Part model, mm, in its own coordinate system. A direction names the side the tool comes from. Round coordinates to 2 decimals unless told otherwise and drop trailing zeros. Write each loop counter-clockwise with the first axis right and the second up, starting at its lowest first coordinate (ties: lowest second). Pieces come first, ordered by that corner, then holes. Notation, with made-up numbers: M 60.5,30.25 L 65.5,30.25 A16 cw 65.5,51.25 Z; hole C -20,49.25 d3. An arc over 180 degrees is marked long. Answer as a JSON object with one key per item and string values. Group by question number.
1. Drop flat-ended pins along their axis: pin 1 (1.5 mm diameter, centred on x = -6, y = -5.5, fed in from +Z); pin 2 (2.5 mm diameter, centred on y = 44.5, z = 10.5, fed in from -X); pin 3 (5 mm diameter, centred on x = -15, z = 10.5, fed in from +Y). Give the stop position or say it passes through.
2. Band-saw the part on B-B, the plane x = -12.25. Write the cut outline in (y, z).
3. Two-plate mould, pull along X, no slides. Class faces 1 (the face through (-17.586, 131.112, 6.409)), 2 (the face through (0.23, 132.16, 6.41)), 3 (the face through (-5.654, 115.116, 6.409)): +X half, -X half, draft (parallel to the pull), parting line (faces both ways), or undercut.
4. Drill centre lines: line 1 (X direction, y = 0.5, z = 6); line 2 (Y direction, x = -5, z = 2.75); line 3 (Y direction, x = -7.25, z = 9.5). Where is each one in solid material? Low to high. Write a range as from..to.
5. Band-saw the part on D-D, the plane y = 104.5. Write the cut outline in (x, z).
6. Band-saw the part on A-A, the plane z = 3. Write the cut outline in (x, y), plus the area to 3 significant figures.
7. Band-saw the part on C-C, the plane y = 13.5. Write the cut outline in (x, z).
8. Which spindle directions (+Z, -Z, +X, -X, +Y, -Y) get a long thin tool onto all of the face, cutting with end or side? Do faces 4 (the face through (-11.556, 158.073, 6.409)), 5 (the face through (-5.439, 87.636, 9.056)), 6 (the face through (-14.329, 36, 6)). Say none if no direction does.
from build123d import *

# Parameters (mm, degrees)
SKETCH1_R      = 2.5
EXTRUDE1_DEPTH = 13
EXTRUDE2_DEPTH = 8


with BuildPart() as part:
    # Sketch1 → Extrude1 (new body)
    with BuildSketch(Plane.XY):
        with BuildLine():
            Line((-14.328597561, 112.637649389), (-14.328597561, -42.362350611))
            ThreePointArc((-14.328597561, -42.362350611), (-5.328597561, -51.362350611), (3.671402439, -42.362350611))
            Line((3.671402439, -42.362350611), (3.671402439, 112.637649389))
            ThreePointArc((3.671402439, 112.637649389), (3.534672216, 114.200482988), (3.128636026, 115.715830679))
            Line((3.128636026, 115.715830679), (-2.753580135, 149.07553625))
            ThreePointArc((-2.753580135, 149.07553625), (-11.753580135, 158.07553625), (-20.753580135, 149.07553625))
            Line((-20.753580135, 149.07553625), (-14.328597561, 112.637649389))
        make_face()
        with Locations((-5.328597561, 112.637649389)):
            Circle(SKETCH1_R, mode=Mode.SUBTRACT)
        with Locations((-5.328597561, -42.362350611)):
            Circle(SKETCH1_R, mode=Mode.SUBTRACT)
        with Locations((-11.753580135, 149.07553625)):
            Circle(SKETCH1_R, mode=Mode.SUBTRACT)
    extrude(amount=EXTRUDE1_DEPTH)

    # Sketch2 → Extrude2 (cut)
    with BuildSketch(Plane.XY.offset(13)):
        with BuildLine():
            Line((-0.328597561, 82.637649389), (-0.328597561, -17.362350611))
            ThreePointArc((-0.328597561, -17.362350611), (-5.328597561, -22.362350611), (-10.328597561, -17.362350611))
            Line((-10.328597561, -17.362350611), (-10.328597561, 82.637649389))
            ThreePointArc((-10.328597561, 82.637649389), (-5.328597561, 87.637649389), (-0.328597561, 82.637649389))
        make_face()
    extrude(amount=-EXTRUDE2_DEPTH, mode=Mode.SUBTRACT)


solid = part.part
Worked answers:
{
 "1": {"pin 1": "stops at z = 5", "pin 2": "stops at x = -14.33", "pin 3": "stops at y = 158.04"},
 "2": {"outline": "M -48.12,0 L 146.63,0 L 146.63,13 L -48.12,13 Z; M 151.53,0 L 158.06,0 L 158.06,13 L 151.53,13 Z"},
 "3": {"face 1": "-X half", "face 2": "+X half", "face 3": "undercut"},
 "4": {"line 1": "x = -14.33..-10.33, -0.33..3.67", "line 2": "y = -51.36..-44.84, -39.88..110.16, 115.12..155.02", "line 3": "y = -51.15..-43.96, -40.76..-21.98, 87.25..111.04, 114.24..156.87"},
 "5": {"outline": "M -14.33,0 L 3.67,0 L 3.67,13 L -14.33,13 Z"},
 "6": {"outline": "M -20.75,149.08 L -14.33,112.64 L -14.33,-42.36 A9 ccw 3.67,-42.36 L 3.67,112.64 A9 ccw 3.13,115.72 L -2.75,149.08 A9 ccw Z; hole C -11.75,149.08 d5; hole C -5.33,-42.36 d5; hole C -5.33,112.64 d5", "area": "3,640 mm^2"},
 "7": {"outline": "M -14.33,0 L 3.67,0 L 3.67,13 L -0.33,13 L -0.33,5 L -10.33,5 L -10.33,13 L -14.33,13 Z"},
 "8": {"face 4": "+Z, -Z, +Y", "face 5": "+Z", "face 6": "+Z, -Z, -X, -Y"}
}
